Geometry check sheet. Reference: the model listing, model coordinates, mm. Face numbers are marked on the shaded views. Coordinates: 2 decimals unless noted, no trailing zeros. Order: outer loops, then holes, each group sorted by start corner. A loop starts at its lowest first (then second) coordinate and runs counter-clockwise, first axis right, second up. Notation, with made-up numbers: (13, -29) - (69, -29) arc R6 ccw to (69, -22) - close; hole circle Ø10 at (62, -14). An arc over 180 degrees is marked (long way). Use CSV: the item, a comma, the result in double quotes. Start each with the question number.
1) Sectioned sample at D-D, the plane z = -11. Record the cut outline in (x, y).
2) Thickness scan on probe 1 along X at (y, z) = (9, -9); probe 2 along Y at (x, z) = (-21, -3); probe 3 along Y at (x, z) = (12.5, 11). Record the ranges inside material, lowest first. Write a range as [from, to].
3) Draft check along X on the marked faces 1, 2, 3 and 4. Enter one of: released by +X, released by -X, zero draft, split by the parting line, or undercut.
4) Depth check by flat-ended pin: P1, Ø3, axis at x = -14, z = -22, coming from the +Y side; P2, Ø1.5, axis at x = -12, y = -3.5, coming from the -Z side; P3, Ø2, axis at x = -6, z = 20.5, coming from the +Y side; P4, Ø7, axis at y = 0, z = 0, coming from the +X side. Enter the tip coordinate at first touch or a pass-through.
5) Sectioned sample at C-C, the plane x = -17.5. Record the cut outline in (y, z).
6) Sectioned sample at A-A, the plane y = 0. Record the cut outline in (x, z), and give its area (3 significant figures).
from build123d import *

# Parameters (mm, degrees)
SKETCH4_R           = 10
BOSS_EXTRUDE2_DEPTH = 8
SKETCH6_R           = 4
CUT_EXTRUDE1_DEPTH  = 38


with BuildPart() as part:
    # Sketch1 → Revolve1 (revolve)
    with BuildSketch(Plane.XY):
        Polygon((12, 35), (15, 35), (15, 0), (-15, 0), (-15, 35), (-12, 35), (-12, 33), (12, 33), align=None)
    revolve(axis=Axis((-15, 0, 0), (1, 0, 0)))

    # Sketch4 → Boss-Extrude2 (add)
    with BuildSketch(Plane.ZY.offset(15)):
        Circle(SKETCH4_R)
    extrude(amount=BOSS_EXTRUDE2_DEPTH)

    # Sketch6 → Cut-Extrude1 (cut)
    with BuildSketch(Plane(origin=(15, 0, 0), x_dir=(0, 0, -1), z_dir=(1, 0, 0))):
        Circle(SKETCH6_R)
    extrude(amount=-CUT_EXTRUDE1_DEPTH, mode=Mode.SUBTRACT)


solid = part.part
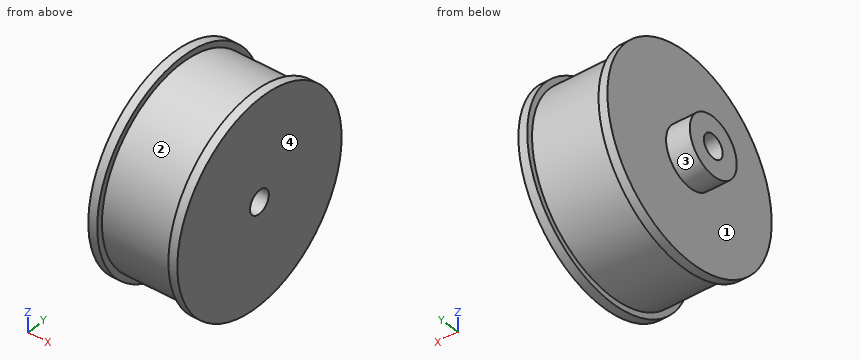
Evaluation:
1,outline,"(-15, -33.23) - (-12, -33.23) - (-12, -31.11) - (12, -31.11) - (12, -33.23) - (15, -33.23) - (15, 33.23) - (12, 33.23) - (12, 31.11) - (-12, 31.11) - (-12, 33.23) - (-15, 33.23) - close"
2,probe 1,"[-15, 15]"
2,probe 2,"[-9.54, -2.65], [2.65, 9.54]"
2,probe 3,"[-33.23, 33.23]"
3,face 1,"released by -X"
3,face 2,"undercut"
3,face 3,"zero draft"
3,face 4,"released by +X"
4,P1,"y = 28.37"
4,P2,"z = -34.89"
4,P3,"y = 26.62"
4,P4,"through"
5,outline,"circle Ø20 at (0, 0); hole circle Ø8 at (0, 0)"
6,outline,"(-23, -10) - (-15, -10) - (-15, -35) - (-12, -35) - (-12, -33) - (12, -33) - (12, -35) - (15, -35) - (15, -4) - (-23, -4) - close; (-23, 4) - (15, 4) - (15, 35) - (12, 35) - (12, 33) - (-12, 33) - (-12, 35) - (-15, 35) - (-15, 10) - (-23, 10) - close"
6,area,"1,860 mm²"
